Design review of the part shown in the three views and the two pictorial views. Dimensions are in mm from the part's minimum x, y and z. A direction names the side the tool comes from. Coordinates: 2 decimals unless noted, no trailing zeros. Loops run counter-clockwise (first coordinate to the right, second up) from the corner with the lowest first, then second, coordinate; pieces in that order, holes last.
Q1. Wall thickness on probe 1 along X at (y, z) = (3.95, 25); probe 2 along Z at (x, y) = (25, 9.4): over which ranges is each line inside the solid? List them lowest first.
Q2. For P1, Ø6, axis at y = 5.5, z = 8.5, coming from the -X side; P2, Ø2, axis at x = 37, y = 7, coming from the -Z side; P3, Ø1, axis at y = 1.5, z = 17, coming from the -X side, all flat-tipped, find the tip position at first contact; note any pin that passes through.
Q3. Machinability: for the marked faces 1 and 2, which of the approach directions +Z, -Z, +X, -X, +Y, -Y give a long, thin tool a straight path to every point of the face, cutting with its end or side? Answer none if there is none.
Q4. Add section C-C on x = 39.5. Give the boundary of the cut face in (y, z).
Q5. Add section A-A on z = 25. Give the boundary of the cut face in (x, y), and give its area (3 significant figures).
Q6. Add section B-B on x = 25. Give the boundary of the cut face in (y, z).
Q7. Draft analysis for pull direction Z (two halves, no side actions). For the marked faces 3, 4, 5 and 6, state which applies: released by +Z, released by -Z, zero draft, split by the parting line, or undercut.
Q8. Add section D-D on y = 2. Give the boundary of the cut face in (x, z), and give its area (3 significant figures).
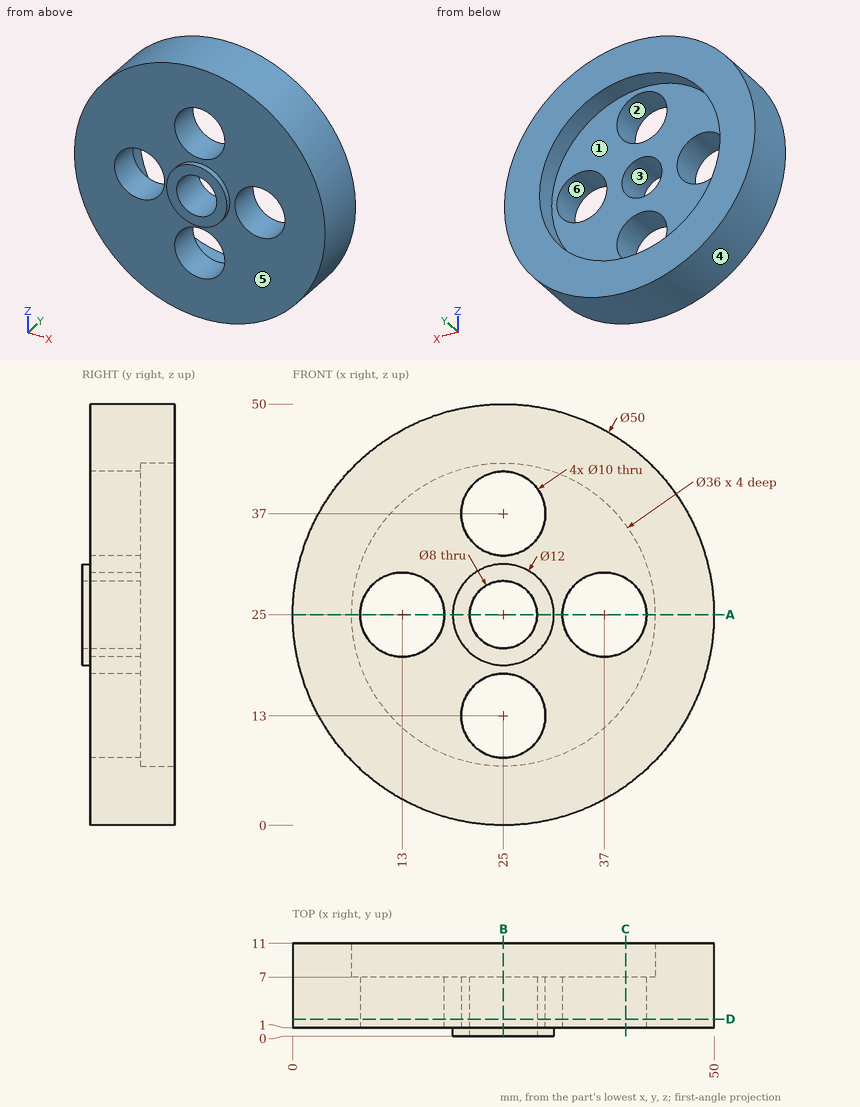
Entries:
1. probe 1: x = 0 to 8, 18 to 21, 29 to 32, 42 to 50
1. probe 2: z = 0 to 7, 43 to 50
2. P1: stops at x = 3.96
2. P2: stops at z = 2.55
2. P3: stops at x = 1.15
3. face 1: +Y
3. face 2: +Y, -Y
4. outline: (1, 4.63) - (11, 4.63) - (11, 14.33) - (7, 14.33) - (7, 20.67) - (1, 20.67) - close; (1, 29.33) - (7, 29.33) - (7, 35.67) - (11, 35.67) - (11, 45.37) - (1, 45.37) - close
5. outline: (0, 1) - (8, 1) - (8, 7) - (7, 7) - (7, 11) - (0, 11) - close; (18, 1) - (19, 1) - (19, 0) - (21, 0) - (21, 7) - (18, 7) - close; (29, 0) - (31, 0) - (31, 1) - (32, 1) - (32, 7) - (29, 7) - close; (42, 1) - (50, 1) - (50, 11) - (43, 11) - (43, 7) - (42, 7) - close
5. area: 192 mm2
6. outline: (0, 19) - (1, 19) - (1, 18) - (7, 18) - (7, 21) - (0, 21) - close; (0, 29) - (7, 29) - (7, 32) - (1, 32) - (1, 31) - (0, 31) - close; (1, 0) - (11, 0) - (11, 7) - (7, 7) - (7, 8) - (1, 8) - close; (1, 42) - (7, 42) - (7, 43) - (11, 43) - (11, 50) - (1, 50) - close
7. face 3: undercut
7. face 4: split by the parting line
7. face 5: zero draft
7. face 6: undercut
8. outline: circle Ø50 at (25, 25); hole circle Ø10 at (13, 25); hole circle Ø10 at (25, 13); hole circle Ø10 at (25, 37); hole circle Ø8 at (25, 25); hole circle Ø10 at (37, 25)
8. area: 1,600 mm2
